```python
from build123d import *

# Parameters (mm, degrees)
SKETCH1_W                = 60
SKETCH1_H                = 20
BASE_DEPTH               = 10
SKETCH2_R                = 3.81
FSR_MOUNT_DEPTH          = 2
CHAMFER1_SIZE            = 2
CHAMFER1_OF_MIRROR1_SIZE = 2
SKETCH5_W                = 40
SKETCH5_H                = 3.5
CUT_EXTRUDE3_DEPTH       = 20
SKETCH6_W                = 40
SKETCH6_H                = 5
BOSS_EXTRUDE4_DEPTH      = 1
SKETCH8_W                = 40
SKETCH8_H                = 5
CUT_EXTRUDE6_DEPTH       = 1
CHAMFER2_SIZE            = 1
SKETCH9_W                = 2
SKETCH9_H                = 8
CUT_EXTRUDE7_DEPTH       = 10
SKETCH10_W               = 60
SKETCH10_H               = 10
CUT_EXTRUDE8_DEPTH       = 1.2
SKETCH11_R               = 1
CUT_EXTRUDE9_DEPTH       = 34.823069051


with BuildPart() as part:
    # Sketch1 → Base (new body)
    with BuildSketch(Plane(origin=(0, 0, 0), x_dir=(1, 0, 0), z_dir=(0, 1, 0))):
        Rectangle(SKETCH1_W, SKETCH1_H)
    extrude(amount=BASE_DEPTH)

    # Sketch2 → FSR Mount (add)
    with BuildSketch(Plane.XZ):
        with Locations(Location((-10, 0, 0), (0, 0, 270))):
            Circle(SKETCH2_R)
    fsr_mount = extrude(amount=FSR_MOUNT_DEPTH)

    # Chamfer1
    chamfer1_edges = [part.edges().sort_by_distance(p)[0] for p in [
        (-10, 0, 3.81),
    ]]
    chamfer(chamfer1_edges, length=CHAMFER1_SIZE - 0.0001)  # a hair under: the kernel refuses the full size

    # Mirror1: FSR Mount across plane
    add(fsr_mount.mirror(Plane(origin=(0, 0, 0), x_dir=(0, 0, 1), z_dir=(1, 0, 0))))

    # Chamfer1 of Mirror1
    chamfer1_of_mirror1_edges = [part.edges().sort_by_distance(p)[0] for p in [
        (10, 0, 3.81),
    ]]
    chamfer(chamfer1_of_mirror1_edges, length=CHAMFER1_OF_MIRROR1_SIZE - 0.0001)  # a hair under: the kernel refuses the full size

    # Sketch5 → Cut-Extrude3 (cut)
    with BuildSketch(Plane(origin=(0, 0, -10), x_dir=(-1, 0, 0), z_dir=(0, 0, -1))):
        with Locations((0, 5)):
            Rectangle(SKETCH5_W, SKETCH5_H)
    extrude(amount=-CUT_EXTRUDE3_DEPTH, mode=Mode.SUBTRACT)

    # Sketch6 → Boss-Extrude4 (add)
    with BuildSketch(Plane(origin=(0, 3.25, 0), x_dir=(1, 0, 0), z_dir=(0, 1, 0))):
        Rectangle(SKETCH6_W, SKETCH6_H)
    extrude(amount=BOSS_EXTRUDE4_DEPTH)

    # Sketch8 → Cut-Extrude6 (cut)
    with BuildSketch(Plane.XZ.offset(-6.75)):
        Rectangle(SKETCH8_W, SKETCH8_H)
    extrude(amount=-CUT_EXTRUDE6_DEPTH, mode=Mode.SUBTRACT)

    # Chamfer2
    chamfer2_edges = [part.edges().sort_by_distance(p)[0] for p in [
        (0, 6.75, -2.5),
        (0, 6.75, 10),
        (0, 3.25, -2.5),
        (0, 3.25, 2.5),
        (0, 3.25, -10),
        (0, 6.75, -10),
        (0, 3.25, 10),
        (0, 6.75, 2.5),
    ]]
    chamfer(chamfer2_edges, length=CHAMFER2_SIZE - 0.0001)  # a hair under: the kernel refuses the full size

    # Sketch9 → Cut-Extrude7 (cut)
    with BuildSketch(Plane.XZ):
        with Locations((-27.5, 0)):
            Rectangle(SKETCH9_W, SKETCH9_H)
    cut_extrude7 = extrude(amount=-CUT_EXTRUDE7_DEPTH, mode=Mode.SUBTRACT)

    # Mirror2: Cut-Extrude7 across plane
    add(cut_extrude7.mirror(Plane(origin=(0, 0, 0), x_dir=(0, 0, 1), z_dir=(1, 0, 0))), mode=Mode.SUBTRACT)

    # Sketch10 → Cut-Extrude8 (cut)
    with BuildSketch(Plane(origin=(0, 10, 0), x_dir=(1, 0, 0), z_dir=(0, 1, 0))):
        Rectangle(SKETCH10_W, SKETCH10_H)
    extrude(amount=-CUT_EXTRUDE8_DEPTH, mode=Mode.SUBTRACT)

    # Sketch11 → Cut-Extrude9 (cut, through all)
    with BuildSketch(Plane(origin=(0, 10, 0), x_dir=(1, 0, 0), z_dir=(0, 1, 0))):
        with Locations(Location((-15, -7.5, 0), (0, 0, 270))):
            Circle(SKETCH11_R)
        with Locations(Location((-5, -7.5, 0), (0, 0, 270))):
            Circle(SKETCH11_R)
        with Locations(Location((5, -7.5, 0), (0, 0, 270))):
            Circle(SKETCH11_R)
        with Locations(Location((15, -7.5, 0), (0, 0, 270))):
            Circle(SKETCH11_R)
    cut_extrude9 = extrude(amount=-CUT_EXTRUDE9_DEPTH, mode=Mode.SUBTRACT)

    # Mirror5: Cut-Extrude9 across plane
    add(cut_extrude9.mirror(Plane.XY), mode=Mode.SUBTRACT)


solid = part.part
```
Design review of the part built by this model. Coordinates are the model's own, in mm. A direction names the side the tool comes from. Round coordinates to 2 decimals unless told otherwise and drop trailing zeros. Write each loop counter-clockwise with the first axis right and the second up, starting at its lowest first coordinate (ties: lowest second). Pieces come first, ordered by that corner, then holes. Notation, with made-up numbers: (61.5, 50.25) -> (110.5, 50.25) arc R21 cw to (110.5, 77.25) -> close; hole circle Ø4 at (45.25, 28.5). An arc over 180 degrees is marked (long way). Write item = value, one per line. Start each with the question number.
1) Tool access review of faces 3 (the face through (0, 0, 0)), 4 (the face through (-0.28, 3.76, 2.99)), 5 (the face through (28, 4, 4)), 6 (the face through (0, 6.75, -6)): name each direction out of +Z, -Z, +X, -X, +Y, -Y from which nothing blocks a thin tool from reaching the whole face with its end or side.
2) Clearance check with flat-ended pins moving along their axes: pin 1 (2.5 mm diameter, centred on x = -5, z = -7.5, fed in from -Y); pin 2 (3 mm diameter, centred on x = 10, z = -6.5, fed in from -Y); pin 3 (3 mm diameter, centred on x = -10, z = 0.5, fed in from +Y). State where each tip first meets the part, or that it passes through.
3) Take a section at B-B, the plane z = -7.5. Count the separate pieces of the cut face and the enclosed holes in it, plus the area to 3 significant figures.
4) Mouldability with a two-part tool opening along X and no side actions: class faces 1 (the face through (-4.01, 1.65, 7.37)), 2 (the face through (0, 10, -8)) as +X half, -X half, draft (parallel to the pull), parting line (faces both ways), or undercut.
5) Wall thickness on probe 1 along X at (y, z) = (1.8, 7.5); probe 2 along X at (y, z) = (1, 2.5); probe 3 along X at (y, z) = (4, -3): over which ranges is each line inside the solid? List them lowest first. Write a range as from..to.
6) Take a section at C-C, the plane x = 25.5. State the section outline as (y, z) points.
Results list:
q1.face_3 = -Y
q1.face_4 = +Z
q1.face_5 = +Y, -Y
q1.face_6 = +Z, -Z
q2.pin_1 = 0
q2.pin_2 = -0.81
q2.pin_3 = 8.8
q3.separate_pieces = 8
q3.enclosed_holes = 0
q3.area = 408 mm²
q4.face_1 = undercut
q4.face_2 = draft
q5.probe_1 = -30..-16, -14..-6, -4..4, 6..14, 16..30
q5.probe_2 = -30..-28.5, -26.5..26.5, 28.5..30
q5.probe_3 = -30..-28.5, -26.5..-20, 20..26.5, 28.5..30
q6.outline = (0, -10) -> (10, -10) -> (10, -5) -> (8.8, -5) -> (8.8, 5) -> (10, 5) -> (10, 10) -> (0, 10) -> close
